Design review of the part built by this model. Coordinates are the model's own, in mm. Coordinates: 2 decimals unless noted, no trailing zeros. Order: outer loops, then holes, each group sorted by start corner. A loop starts at its lowest first (then second) coordinate and runs counter-clockwise, first axis right, second up. Notation, with made-up numbers: (53, 7.25) -> (109, 7.25) arc R28 cw to (109, 27.25) -> close; hole circle Ø3 at (12, 17.25). An arc over 180 degrees is marked (long way). Write item = value, one per line.
```python
from build123d import *

# Parameters (mm, degrees)
ESTRUSIONE_ESTRUSIONE1_DEPTH = 18
TAGLIO_ESTRUSIONE3_DEPTH     = 61
TAGLIO_ESTRUSIONE5_DEPTH     = 100


with BuildPart() as part:
    # Schizzo1 → Estrusione-Estrusione1 (new body)
    with BuildSketch(Plane.XY):
        with BuildLine():
            Line((-452.35, 100), (-464, 100))
            Line((-464, 100), (-464, 0))
            Line((-464, 0), (0, 0))
            Line((0, 0), (0, 100))
            Line((0, 100), (-11.650000002, 100))
            ThreePointArc((-11.650000002, 100), (-14.825000002, 96.825), (-18.000000001, 100))
            Line((-18.000000001, 100), (-18.000000001, 118.000682307))
            ThreePointArc((-18.000000001, 118.000682307), (-14.824658921, 121.174999982), (-11.650000075, 118))
            Line((-11.650000075, 118), (18, 118))
            Line((18, 118), (18, 318))
            Line((18, 318), (-482, 318))
            Line((-482, 318), (-482, 118))
            Line((-482, 118), (-452.35, 118))
            ThreePointArc((-452.35, 118), (-449.175, 121.175), (-446, 118))
            Line((-446, 118), (-446, 100))
            ThreePointArc((-446, 100), (-449.175, 96.825), (-452.35, 100))
        make_face()
    extrude(amount=ESTRUSIONE_ESTRUSIONE1_DEPTH)

    # Schizzo1<6> → Taglio-Estrusione3 (cut)
    with BuildSketch(Plane.XY):
        with BuildLine():
            Line((-399.65, 118), (-64.349999981, 118))
            ThreePointArc((-64.349999981, 118), (-61.175172814, 121.174999995), (-58, 118.000345666))
            Line((-58, 118.000345666), (-58, 100.000682304))
            ThreePointArc((-58, 100.000682304), (-61.174658811, 96.825341189), (-64.349999927, 100))
            Line((-64.349999927, 100), (-399.65, 100))
            ThreePointArc((-399.65, 100), (-402.825, 96.825), (-406, 100))
            Line((-406, 100), (-406, 118))
            ThreePointArc((-406, 118), (-402.825, 121.175), (-399.65, 118))
        make_face()
    extrude(amount=TAGLIO_ESTRUSIONE3_DEPTH, mode=Mode.SUBTRACT)

    # Schizzo1<8> → Taglio-Estrusione5 (cut)
    with BuildSketch(Plane.XY):
        with BuildLine():
            Line((-412.05, 185.92), (-433.05, 185.92))
            ThreePointArc((-433.05, 185.92), (-436.225, 189.095), (-433.05, 192.27))
            Line((-433.05, 192.27), (-433.05, 197.57))
            ThreePointArc((-433.05, 197.57), (-436.225, 200.745), (-433.05, 203.92))
            Line((-433.05, 203.92), (-412.05, 203.92))
            Line((-412.05, 203.92), (-412.05, 224.92))
            ThreePointArc((-412.05, 224.92), (-408.875, 228.095), (-405.7, 224.92))
            Line((-405.7, 224.92), (-400.4, 224.92))
            ThreePointArc((-400.4, 224.92), (-397.225, 228.095), (-394.05, 224.92))
            Line((-394.05, 224.92), (-394.05, 203.92))
            Line((-394.05, 203.92), (-373.05, 203.92))
            ThreePointArc((-373.05, 203.92), (-369.875, 200.745), (-373.05, 197.57))
            Line((-373.05, 197.57), (-373.05, 192.27))
            ThreePointArc((-373.05, 192.27), (-369.875, 189.095), (-373.05, 185.92))
            Line((-373.05, 185.92), (-394.05, 185.92))
            Line((-394.05, 185.92), (-394.05, 164.92))
            ThreePointArc((-394.05, 164.92), (-397.225, 161.745), (-400.4, 164.92))
            Line((-400.4, 164.92), (-405.7, 164.92))
            ThreePointArc((-405.7, 164.92), (-408.875, 161.745), (-412.05, 164.92))
            Line((-412.05, 164.92), (-412.05, 185.92))
        make_face()
    extrude(amount=TAGLIO_ESTRUSIONE5_DEPTH, mode=Mode.SUBTRACT)


solid = part.part
```
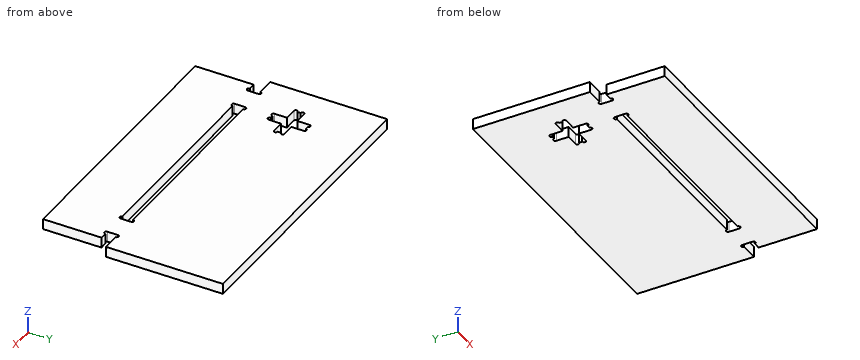
(1) Insertion check: pin 1 (1 mm diameter, centred on y = 97.5, z = 6.5, fed in from -X); pin 2 (9 mm diameter, centred on y = 107, z = 4.5, fed in from -X); pin 3 (9 mm diameter, centred on y = 64, z = 11, fed in from +X). Each pin has a flat end and moves straight along its axis. Give the tip position at first contact, or say it passes through.
Report:
pin_1 = -464
pin_2 = -446
pin_3 = 0
(2) We need section B-B (y = 220). Write out the cut boundary in (x, z).
Report:
outline = (-482, 0) -> (-412.05, 0) -> (-412.05, 18) -> (-482, 18) -> close; (-394.05, 0) -> (18, 0) -> (18, 18) -> (-394.05, 18) -> close
(3) For L1, parallel to Y at x = -70.5, z = 7.5; L2, parallel to Y at x = -415.5, z = 13.25; L3, parallel to Y at x = -393, z = 15.5, list the stretches that pass through material, from the lowest coordinate up.
Report:
L1 = 0 to 100, 118 to 318
L2 = 0 to 185.92, 203.92 to 318
L3 = 0 to 100, 118 to 185.92, 203.92 to 318
(4) We need section D-D (y = 22.5). Write out the cut boundary in (x, z).
Report:
outline = (-464, 0) -> (0, 0) -> (0, 18) -> (-464, 18) -> close
(5) We need section C-C (z = 15). Give the number of separate pieces and of enclosed holes in the cut face, and give its area (3 significant figures).
Report:
separate_pieces = 1
enclosed_holes = 2
area = 146,000 mm²
(6) We need section A-A (x = -139.5). Write out the cut boundary in (y, z).
Report:
outline = (0, 0) -> (100, 0) -> (100, 18) -> (0, 18) -> close; (118, 0) -> (318, 0) -> (318, 18) -> (118, 18) -> close
